from build123d import *

# Parameters (mm, degrees)
F4_DEPTH = 4.572
F4_TAPER = 15


with BuildPart() as f1:
    # F0 (on Front) → F1 (revolve)
    with BuildSketch(Plane.XZ):
        with BuildLine():
            Line((-6.858, 12.7), (-10.033, 12.7))
            Line((-10.033, 12.7), (-10.033, -4.572))
            Line((-10.033, -4.572), (-10.9982, -4.572))
            ThreePointArc((-10.9982, -4.572), (-12.7421516444, -9.1602447444), (-13.335, -14.0328095721))
            ThreePointArc((-13.335, -14.0328095721), (-12.7463257854, -18.8884436966), (-11.0144111466, -23.4627405568))
            ThreePointArc((-11.0144111466, -23.4627405568), (-8.4355524205, -29.6589038682), (-6.9839312526, -36.2114413992))
            ThreePointArc((-6.9839312526, -36.2114413992), (-6.9417882519, -36.290438613), (-6.858, -36.322))
            Line((-6.858, -36.322), (-6.858, 12.7))
        make_face()
    revolve(axis=Axis((-6.858, 0, -6.3344838709), (0, 0, -1)))


with BuildPart() as f2_1:
    # F2: instance of F1
    add(f1.part.mirror(Plane.YZ))


with BuildPart() as f1_1:
    add(f1.part)

    add(f2_1.part)  # F4 merges F2_1
    # F3 (on face) → F4 (join)
    with BuildSketch(Plane.XY.offset(-4.572)):
        with BuildLine():
            ThreePointArc((3.429, 3.8507606314), (0, 2.5453212627), (-3.429, 3.8507606314))
            ThreePointArc((-3.429, 3.8507606314), (-12.0142, 0), (-3.429, -3.8507606314))
            ThreePointArc((-3.429, -3.8507606314), (0, -2.5453212627), (3.429, -3.8507606314))
            ThreePointArc((3.429, -3.8507606314), (12.0142, 0), (3.429, 3.8507606314))
        make_face()
    extrude(amount=F4_DEPTH, taper=F4_TAPER)


solid = f1_1.part
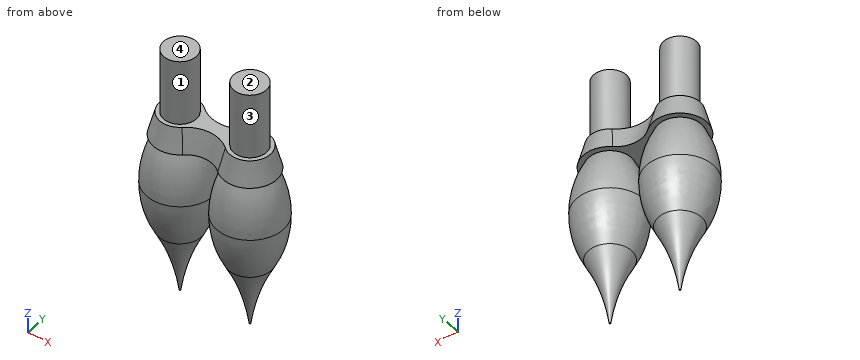
The model under review builds one solid part; all positions refer to its coordinate system, in mm. Face numbers are marked on the shaded views. A direction names the side the tool comes from. Give positions to 0.01 mm unless a question says otherwise; leave off trailing zeros. Loops run counter-clockwise (first coordinate to the right, second up) from the corner with the lowest first, then second, coordinate; pieces in that order, holes last. Notation, with made-up numbers: (62, 3.25) -> (103, 3.25) arc R8 ccw to (103, 13.25) -> close; hole circle Ø11 at (50.5, -14). An arc over 180 degrees is marked (long way). Put each result on its own line as item: value. Start each with the question number.
1. Wall thickness on probe 1 along X at (y, z) = (-3.25, -6.5); probe 2 along X at (y, z) = (3.25, -2); probe 3 along Z at (x, y) = (2.5, -1.5): over which ranges is each line inside the solid? List them lowest first.
2. Clearance check with flat-ended pins moving along their axes: P1, Ø1.5, axis at y = 5, z = -5.5, coming from the -X side; P2, Ø3, axis at x = 5, z = -1, coming from the +Y side; P3, Ø10, axis at x = 10, z = -28.5, coming from the -Y side. State where each tip first meets the part, or that it passes through.
3. We need section A-A on z = 8. State the section outline as (x, y) points (3 decimals).
4. For the marked faces 1 and 2, list the 3-axis set-ups (+Z, -Z, +X, -X, +Y, -Y) from which the entire face can be reached by the end or side of a thin tool; tool diameter is ignored.
5. Mouldability with a two-part tool opening along X and no side actions: class the marked faces 3 and 4 as released by +X, released by -X, zero draft, split by the parting line, or undercut.
Determined:
1. probe 1: -10.7 to -3.02, 3.02 to 10.7
1. probe 2: -9.92 to -3.79, 3.79 to 9.92
1. probe 3: -22.54 to -5.52, -4.57 to 0
2. P1: x = -8.81
2. P2: y = 4.42
2. P3: y = -3.76
3. outline: circle Ø6.35 at (-6.858, 0); circle Ø6.35 at (6.858, 0)
4. face 1: +Z
4. face 2: +Z, +X, -X, +Y, -Y
5. face 3: undercut
5. face 4: zero draft
